Design review of the part built by this model. Coordinates are the model's own, in mm. A direction names the side the tool comes from. Give positions to 0.01 mm unless a question says otherwise; leave off trailing zeros. Write each loop counter-clockwise with the first axis right and the second up, starting at its lowest first coordinate (ties: lowest second). Pieces come first, ordered by that corner, then holes. Notation, with made-up numbers: (-22, 39) - (-2, 39) arc R12 cw to (-2, 52) - close; hole circle Ø1 at (81.5, 32). An arc over 180 degrees is marked (long way). Use a Markdown table: item, result. Add a question column.
Autodesk Inventor part; units mm, degrees
ref_plane "YZ Plane" through (0, 0, 0) normal (1, 0, 0) x (0, 1, 0)
ref_plane "XZ Plane" through (0, 0, 0) normal (0, 1, 0) x (-1, 0, 0)
ref_plane "XY Plane" through (0, 0, 0) normal (0, 0, 1) x (1, 0, 0)
sketch "Skizze1" plane through (0, 0, 0) normal (0, 0, 1) x (1, 0, 0)
  line L0 (-34.2467, 13.3525) -> (-93.0967, 13.3525)
  line L1 (-93.0967, 13.3525) -> (-93.0967, 100.3525)
  line L2 (-93.0967, 100.3525) -> (-34.2467, 100.3525)
  line L3 (-34.2467, 100.3525) -> (-34.2467, 13.3525)
  point P0 (0, 0)
  dimension "d0" = 58.85
  dimension "d1" = 87
extrude "Extrusion1" add sketch "Skizze1" along normal blind 3.5
sketch "Skizze2" plane through (0, 0, 3.5) normal (0, 0, 1) x (1, 0, 0)
  line L0 (-93.0967, 13.3525) -> (-34.2467, 13.3525)
  line L1 (-93.0967, 13.3525) -> (-96.5967, 13.3525)
  line L2 (-96.5967, 13.3525) -> (-96.5967, 103.8525)
  line L3 (-96.5967, 103.8525) -> (-30.7467, 103.8525)
  line L4 (-34.2467, 100.3525) -> (-93.0967, 100.3525)
  line L5 (-30.7467, 103.8525) -> (-30.7467, 13.3525)
  line L6 (-30.7467, 13.3525) -> (-34.2467, 13.3525)
  line L7 (-34.2467, 13.3525) -> (-34.2467, 100.3525)
  line L8 (-34.2467, 13.3525) -> (-34.2467, 100.3525)
  line L9 (-34.2467, 100.3525) -> (-93.0967, 100.3525)
  line L10 (-93.0967, 100.3525) -> (-93.0967, 13.3525)
  line L11 (-30.7467, 13.3525) -> (-30.7467, 9.8525)
  line L12 (-30.7467, 9.8525) -> (-96.5967, 9.8525)
  line L13 (-96.5967, 9.8525) -> (-96.5967, 13.3525)
  line L14 (-30.7467, 13.3525) -> (-96.5967, 13.3525)
  point P0 (0, 0)
  dimension "d4" = 3.5
  dimension "d5" = 3.5
  dimension "d6" = 3.5
  dimension "d7" = 3.5
extrude "Extrusion2" add sketch "Skizze2" against normal blind 5.6 contours L0 L6 L11 L12 L13 L1
sketch "Skizze3" plane through (0, 0, 0) normal (0, 0, -1) x (-1, 0, 0)
  line L0 (30.7467, 15.473) -> (30.7467, 103.8525)
  line L1 (30.7467, 103.8525) -> (96.5967, 103.8525)
  line L2 (34.2467, 100.3525) -> (93.0967, 100.3525)
  line L3 (96.5967, 103.8525) -> (96.5967, 13.3525)
  line L4 (93.0967, 100.3525) -> (93.0967, 13.3525)
  line L5 (34.2467, 100.3525) -> (34.2467, 13.3525)
  line L6 (30.7467, 13.3525) -> (30.7467, 15.473)
  line L7 (30.7467, 13.3525) -> (34.2467, 13.3525)
  line L8 (30.7467, 13.3525) -> (34.2467, 13.3525)
  line L9 (34.2467, 13.3525) -> (34.2467, 100.3525)
  line L10 (34.2467, 13.3525) -> (34.2467, 100.3525)
  line L11 (34.2467, 100.3525) -> (93.0967, 100.3525)
  line L12 (34.2467, 13.3525) -> (93.0967, 13.3525)
  line L13 (93.0967, 13.3525) -> (96.5967, 13.3525)
  line L14 (93.0967, 13.3525) -> (96.5967, 13.3525)
  line L15 (96.5967, 13.3525) -> (96.5967, 103.8525)
  point P0 (0, 0)
  dimension "d10" = 3.5
  dimension "d11" = 3.5
  dimension "d12" = 3.5
extrude "Extrusion3" add sketch "Skizze3" along normal blind 4.1 contours L0 L1 L3 L13 L4 L2 L5 L7 L6
sketch "Skizze4" plane through (0, 0, 0) normal (0, 0, 1) x (1, 0, 0)
  line L0 (-34.2467, 13.3525) -> (-93.0967, 13.3525)
  line L1 (-96.5967, 9.8525) -> (-96.5967, 13.3525)
  line L2 (-93.0967, 13.3525) -> (-96.5967, 13.3525)
  line L3 (-96.5967, 103.8525) -> (-30.7467, 103.8525)
  line L4 (-96.5967, 13.3525) -> (-96.5967, 103.8525)
  line L5 (-96.5967, 103.8525) -> (-30.7467, 103.8525)
  line L6 (-30.7467, 103.8525) -> (-30.7467, 13.3525)
  line L7 (-30.7467, 103.8525) -> (-30.7467, 13.3525)
  line L8 (-34.2467, 100.3525) -> (-34.2467, 13.3525)
  line L9 (-30.7467, 13.3525) -> (-34.2467, 13.3525)
  line L10 (-34.2467, 100.3525) -> (-93.0967, 100.3525)
  line L11 (-34.2467, 13.3525) -> (-34.2467, 100.3525)
  line L12 (-34.2467, 100.3525) -> (-93.0967, 100.3525)
  line L13 (-93.0967, 100.3525) -> (-93.0967, 13.3525)
  point P0 (0, 0)
extrude "Extrusion4" add sketch "Skizze4" along normal blind 3.5 contours L8 L10 L13 L2 L4 L3 L6 L9
sketch "Skizze5" plane through (-96.5967, 103.8525, -4.1) normal (0, 1, 0) x (1, 0, 0)
  line L0 (62.35, 0) -> (3.5, 0)
  line L1 (24.85, 0) -> (41.85, 0)
  line L2 (41.85, 0) -> (41.85, -2)
  line L3 (41.85, -2) -> (24.85, -2)
  line L4 (24.85, -2) -> (24.85, 0)
  line L5 (65.85, -7.6) -> (65.85, 0)
  line L6 (0, -7.6) -> (0, 0)
  point P0 (96.5967, -4.1)
  dimension "d17" = 17
  dimension "d18" = 24
  dimension "d19" = 2
  dimension "d40" = 24.85
extrude "Extrusion5" cut sketch "Skizze5" against normal blind 3.5
sketch "Skizze7" plane through (0, 0, -4.1) normal (0, 0, -1) x (-1, 0, 0)
  line L0 (30.7467, 9.8525) -> (30.7467, 103.8525)
  line L1 (30.7467, 9.8525) -> (96.5967, 9.8525)
  line L2 (96.5967, 13.3525) -> (96.5967, 103.8525)
  arc A0 (96.5967, 83.3525) -> (96.5967, 98.3525) centre (96.5967, 90.8525) ccw
  line L3 (96.5967, 103.8525) -> (71.7467, 103.8525)
  point P0 (0, 0)
  point P1 (30.7467, 15.3525)
  point P2 (30.7467, 30.3525)
  dimension "d24" = 15
  dimension "d25" = 13
sketch "Skizze8" plane through (-30.7467, 9.8525, 3.5) normal (1, 0, 0) x (0, 0, -1)
  point P0 (3.5, -9.8525)
extrude "Extrusion6" [suppressed]
sketch "Skizze9" plane through (0, 0, -4.1) normal (0, 0, -1) x (-1, 0, 0)
  circle A0 centre (27.7467, 22.8525) radius 2
  line L0 (30.7467, 103.8525) -> (30.7467, 13.3525)
  point P0 (0, 0)
  point P1 (30.7467, 22.8525)
  point P2 (30.7467, 15.3525)
  dimension "d28" = 7.5
  dimension "d29" = 4
  dimension "d30" = 3
extrude "Extrusion7" cut sketch "Skizze9" against normal through all
sketch "Skizze10" plane through (0, 0, -4.1) normal (0, 0, -1) x (-1, 0, 0)
  circle A0 centre (99.5967, 90.8525) radius 2
  line L0 (96.5967, 13.3525) -> (96.5967, 103.8525)
  point P0 (0, 0)
  point P1 (96.5967, 98.3525)
  dimension "d33" = 4
  dimension "d34" = 3
extrude "Extrusion8" cut sketch "Skizze10" against normal through all
sketch "Skizze11" plane through (0, 0, 3.5) normal (0, 0, 1) x (1, 0, 0)
  point P0 (0, 0)
sketch "Skizze12" plane through (-30.7467, 9.8525, 3.5) normal (1, 0, 0) x (0, 0, -1)
  line L0 (7.6, 3.5) -> (7.6, 94)
  line L1 (7.6, 3.5) -> (0, 3.5)
  line L2 (0, 3.5) -> (0, 0)
  line L3 (0, 0) -> (7.6, 0)
  line L4 (7.6, 0) -> (7.6, 3.5)
  point P0 (3.5, -9.8525)
extrude "Extrusion9" cut sketch "Skizze12" against normal through all
sketch "Skizze13" plane through (-30.7467, 13.3525, 3.5) normal (1, 0, 0) x (0, 0, -1)
  line L0 (7.6, 87) -> (7.6, 0)
  line L1 (7.6, 0) -> (5.1687, 0)
  line L2 (5.1687, 0) -> (5.1687, 2.037)
  line L3 (5.1687, 2.037) -> (7.6, 2.037)
  line L4 (7.6, 2.037) -> (7.6, 0)
  point P0 (3.5, -13.3525)
sketch "Skizze14" plane through (0, 0, 3.5) normal (0, 0, 1) x (1, 0, 0)
  line L0 (-30.7467, 103.8525) -> (-30.7467, 13.3525)
  arc A0 (-30.7467, 18.8525) -> (-30.7467, 33.8525) centre (-30.7467, 26.3525) ccw
  line L1 (-96.5967, 103.8525) -> (-96.5967, 13.3525)
  arc A1 (-96.5967, 98.3525) -> (-96.5967, 83.3525) centre (-96.5967, 90.8525) ccw
  line L2 (-96.5967, 13.3525) -> (-30.7467, 13.3525)
  circle A2 centre (-27.7467, 26.3525) radius 2
  circle A3 centre (-99.5967, 90.8525) radius 2
  point P0 (0, 0)
  dimension "d41" = 15
  dimension "d42" = 15
  dimension "d43" = 13
  dimension "d44" = 13
  dimension "d45" = 3
  dimension "d46" = 4
  dimension "d47" = 3
  dimension "d48" = 4
sketch "Skizze15" plane through (-96.5967, 13.3525, 3.5) normal (-1, 0, 0) x (0, 0, 1)
  point P0 (-3.5, -13.3525)
extrude "Extrusion10" add sketch "Skizze14" against normal blind 7.6
sketch "Skizze16" plane through (-93.0967, 13.3525, 0) normal (0, -1, 0) x (1, 0, 0)
  point P0 (93.0967, 0)
sketch "Skizze17" plane through (0, 0, 3.5) normal (0, 0, 1) x (1, 0, 0)
  line L0 (-13.2494, 3.641) -> (-122.0727, 3.641)
  line L1 (-122.0727, 3.641) -> (-122.0727, 119.9278)
  line L2 (-122.0727, 119.9278) -> (-13.2494, 119.9278)
  line L3 (-13.2494, 119.9278) -> (-13.2494, 3.641)
  point P0 (0, 0)
extrude "Extrusion11" cut sketch "Skizze17" against normal blind 1
sketch "Skizze18" plane through (0, 0, 0) normal (0, 0, -1) x (-1, 0, 0)
  point P0 (0, 0)
ref_plane "Arbeitsebene1" through (-96.5967, 103.8525, -4.1) normal (0, 1, 0) x (1, 0, 0)
sketch "Skizze19" plane through (-96.5967, 103.8525, -4.1) normal (0, 1, 0) x (1, 0, 0)
  line L0 (0, -6.6) -> (0, 0)
  line L1 (0, 0) -> (24.85, 0)
  line L2 (0, -6.6) -> (65.85, -6.6)
  line L3 (65.85, -6.6) -> (65.85, 0)
  line L4 (41.85, 0) -> (65.85, 0)
  line L5 (24, -2) -> (41.85, -2)
  line L6 (41.85, -2) -> (41.85, 5.2977)
  line L7 (41.85, 5.2977) -> (24, 5.2977)
  line L8 (24, 5.2977) -> (24, -2)
  point P0 (96.5967, -4.1)
  dimension "d54" = 24
  dimension "d55" = 24
  dimension "d56" = 2
extrude "Extrusion12" cut sketch "Skizze19" against normal blind 10 contours L8 L7 L6 L5
properties part number "Unterteil_fertig2"
(1) Mouldability with a two-part tool opening along Y and no side actions: class faces 1 (the face through (-28.007, 28.335, -0.754)), 2 (the face through (-104.095, 91.017, -0.754)), 3 (the face through (-98.52, 92.54, -0.75)), 4 (the face through (-63.3, 100.352, -1.6)) as +Y half, -Y half, draft (parallel to the pull), parting line (faces both ways), or undercut.
(2) Insertion check: pin 1 (5 mm diameter, centred on x = -89, y = 74, fed in from -Z); pin 2 (2 mm diameter, centred on y = 102.5, z = -3.5, fed in from +X); pin 3 (5 mm diameter, centred on x = -27.75, y = 26.35, fed in from +Z); pin 4 (3 mm diameter, centred on y = 102, z = 0.5, fed in from -X). Each pin has a flat end and moves straight along its axis. Give the tip position at first contact, or say it passes through.
(3) Add section A-A (y = 39). State the section outline as (x, z) points, and give its area (3 significant figures).
(4) For line 1 along X through (y, z) = (91.5, -1); line 2 along X through (y, z) = (69.5, -2.5); line 3 along X through (y, z) = (17.5, 1.75), list the stretches that pass through material, from the lowest coordinate up.
(5) Add section C-C (y = 87). State the section outline as (x, z) points, and give its area (3 significant figures).
(6) Tool access review of faces 5 (the face through (-96.597, 48, -1)), 6 (the face through (-54.747, 102, -3)), 7 (the face through (-30.747, 69, -1)), 8 (the face through (-64, 57, 0)), 9 (the face through (-96.597, 101, -1)): name each direction out of +Z, -Z, +X, -X, +Y, -Y from which nothing blocks a thin tool from reaching the whole face with its end or side.
(7) Add section D-D (x = -71). State the section outline as (y, z) points.
(8) Add section B-B (x = -50). State the section outline as (y, z) points, and give its area (3 significant figures).
Answers follow:
| question | item | result |
|---|---|---|
| 1 | face 1 | undercut |
| 1 | face 2 | parting line |
| 1 | face 3 | undercut |
| 1 | face 4 | -Y half |
| 2 | pin 1 | z = 0 |
| 2 | pin 2 | x = -30.75 |
| 2 | pin 3 | z = 2.5 |
| 2 | pin 4 | x = -96.6 |
| 3 | outline | (-96.6, -4.1) - (-93.1, -4.1) - (-93.1, 0) - (-34.25, 0) - (-34.25, -4.1) - (-30.75, -4.1) - (-30.75, 2.5) - (-96.6, 2.5) - close |
| 3 | area | 193 mm^2 |
| 4 | line 1 | -104.07 to -101.49, -97.7 to -93.1, -34.25 to -30.75 |
| 4 | line 2 | -96.6 to -93.1, -34.25 to -30.75 |
| 4 | line 3 | -96.6 to -30.75 |
| 5 | outline | (-103.03, -4.1) - (-93.1, -4.1) - (-93.1, 0) - (-34.25, 0) - (-34.25, -4.1) - (-30.75, -4.1) - (-30.75, 2.5) - (-103.03, 2.5) - close |
| 5 | area | 236 mm^2 |
| 6 | face 5 | +Z, -Z, -X, -Y |
| 6 | face 6 | -Z, +Y, -Y |
| 6 | face 7 | +Z, -Z, +X, +Y |
| 6 | face 8 | -Z, -Y |
| 6 | face 9 | +Z, -Z, -X, +Y |
| 7 | outline | (13.35, 0) - (100.35, 0) - (100.35, -2.1) - (103.85, -2.1) - (103.85, 2.5) - (13.35, 2.5) - close |
| 8 | outline | (13.35, 0) - (100.35, 0) - (100.35, -4.1) - (103.85, -4.1) - (103.85, 2.5) - (13.35, 2.5) - close |
| 8 | area | 241 mm^2 |
